```python
from build123d import *

# Parameters (mm, degrees)
RESSALTO_EXTRUS_O1_DEPTH   = 10
ESBO_O2_W                  = 10
ESBO_O2_H                  = 10
ESBO_O2_W_2                = 210
ESBO_O2_H_2                = 220
RESSALTO_EXTRUS_O4_DEPTH   = 50
ESBO_O7_R                  = 40
CORTE_EXTRUS_O1_DEPTH      = 3
ESBO_O21_W                 = 200
ESBO_O21_H                 = 25
CORTE_EXTRUS_O5_DEPTH      = 100
CORTE_EXTRUS_O6_DEPTH      = 161.25
CORTE_EXTRUS_O6_DEPTH_BACK = 1.25
ESBO_O23_W                 = 150
ESBO_O23_H                 = 5
RESSALTO_EXTRUS_O5_DEPTH   = 70


with BuildPart() as part:
    # Esboço1 → Ressalto-extrusão1 (new body)
    with BuildSketch(Plane.XY):
        Polygon((-99.217703787, 25.02394247), (70.782296213, 25.02394247), (70.782296213, 0), (70.782296213, -214.97605753), (-99.217703787, -214.97605753), (-269.217703787, -214.97605753), (-269.217703787, 0), (-269.217703787, 25.02394247), align=None)
    extrude(amount=RESSALTO_EXTRUS_O1_DEPTH)

    # Esboço2 → Ressalto-extrusão4 (add)
    with BuildSketch(Plane.XY.offset(10)):
        with Locations((-54.217703787, -209.97605753)):
            Rectangle(ESBO_O2_W, ESBO_O2_H)
        with Locations((-164.217703787, -209.97605753)):
            Rectangle(ESBO_O2_W_2, ESBO_O2_H)
        with Locations((-54.217703787, -94.97605753)):
            Rectangle(ESBO_O2_W, ESBO_O2_H_2)
        Polygon((-59.217703787, 15.02394247), (-49.217703787, 15.02394247), (-49.217703787, 25.02394247), (-269.217703787, 25.02394247), (-269.217703787, 15.02394247), align=None)
    extrude(amount=RESSALTO_EXTRUS_O4_DEPTH)

    # Esboço7 → Corte-extrusão1 (cut)
    with BuildSketch(Plane.XY.offset(10)):
        with Locations((10.782296213, -154.97605753)):
            Circle(ESBO_O7_R)
    extrude(amount=-CORTE_EXTRUS_O1_DEPTH, mode=Mode.SUBTRACT)

    # Esboço21 → Corte-extrusão5 (cut)
    with BuildSketch(Plane(origin=(0, 25.02394247, 0), x_dir=(1, 0, 0), z_dir=(0, 1, 0))):
        with Locations((-159.217703787, -37.5)):
            Rectangle(ESBO_O21_W, ESBO_O21_H)
    extrude(amount=-CORTE_EXTRUS_O5_DEPTH, mode=Mode.SUBTRACT)

    # Esboço23 → Corte-extrusão6 (cut, two sides: drawn at the far end of the back side and taken through both)
    with BuildSketch(Plane.XZ.offset(-15.02394247).offset(-CORTE_EXTRUS_O6_DEPTH_BACK)):
        with Locations((-194.217703787, 55)):
            Rectangle(ESBO_O23_W, ESBO_O23_H)
    extrude(amount=CORTE_EXTRUS_O6_DEPTH + CORTE_EXTRUS_O6_DEPTH_BACK, mode=Mode.SUBTRACT)

    # Esboço28 → Ressalto-extrusão5 (add)
    with BuildSketch(Plane.XY.offset(10)):
        Polygon((70.782296213, -84.97605753), (70.782296213, 25.02394247), (60.782296213, 25.02394247), (-39.217703787, 25.02394247), (-49.217703787, 25.02394247), (-49.217703787, -74.97605753), (-49.217703787, -84.97605753), align=None)
    extrude(amount=RESSALTO_EXTRUS_O5_DEPTH)


solid = part.part
```
Geometry check sheet. Reference: the model listing, model coordinates, mm. A direction names the side the tool comes from. Round coordinates to 2 decimals unless told otherwise and drop trailing zeros. Order: outer loops, then holes, each group sorted by start corner. A loop starts at its lowest first (then second) coordinate and runs counter-clockwise, first axis right, second up. Notation, with made-up numbers: M 39.25,61 L 69.25,61 A25 ccw 69.25,94 Z; hole C 79.25,28 d5. An arc over 180 degrees is marked long. Write item = value, one per line.
Q1. Release check for a two-part mould opening along X. For faces 6 (the flat face through (38, -120, 10)), 7 (the flat face through (-259.218, 20, 38)), 8 (the flat face through (-49.218, -29, 70)), 9 (the flat face through (10, -154, 7)) record: released by +X, released by -X, zero draft, split by the parting line, or undercut.
Answer block:
face_6 = zero draft
face_7 = undercut
face_8 = released by -X
face_9 = undercut
Q2. Set-up check for faces 1 (the flat face through (-163, -204.976, 35)), 2 (the flat face through (-49.218, -151, 35)), 3 (the cylindrical face through (5.575, -115.316, 8.521)), 4 (the flat face through (-161, 20, 50)), 5 (the flat face through (-54, -94, 60)): record each of +Z, -Z, +X, -X, +Y, -Y from which the full face is reachable in a straight line by a thin tool's end or side.
Answer block:
face_1 = +Z, -X
face_2 = +Z, +X, -Y
face_3 = +Z
face_4 = +Y
face_5 = +Z, -X, +Y, -Y
Q3. Scan lines: line 1 (Y direction, x = -135, z = 52); line 2 (Z direction, x = -44, y = -148.5); line 3 (X direction, y = -156, z = 21). Record each from-to range of solid material in increasing order.
Answer block:
line_1 = -214.98 to -204.98, 15.02 to 25.02
line_2 = 0 to 10
line_3 = -59.22 to -49.22
Q4. Section check A-A (z = 41). Enter the section's corners in (x, y), plus the area to 3 significant figures.
Answer block:
outline = M -269.22,-214.98 L -49.22,-214.98 L -49.22,-84.98 L 70.78,-84.98 L 70.78,25.02 L -59.22,25.02 L -59.22,-204.98 L -269.22,-204.98 Z; M -269.22,15.02 L -259.22,15.02 L -259.22,25.02 L -269.22,25.02 Z
area = 17,800 mm^2
Q5. Depth check by flat-ended pin: pin 1 Ø1 at (x, y) = (-201.5, 16) entering from +Z; pin 2 Ø2 at (y, z) = (-24.5, 32) entering from -X; pin 3 Ø25 at (y, z) = (-178, 29) entering from +X. Enter the tip coordinate at first touch or a pass-through.
Answer block:
pin_1 = 60
pin_2 = -59.22
pin_3 = -49.22
Q6. Section check B-B (x = -94.5). Enter the section's corners in (y, z), plus the area to 3 significant figures.
Answer block:
outline = M -214.98,0 L 25.02,0 L 25.02,25 L 15.02,25 L 15.02,10 L -204.98,10 L -204.98,60 L -214.98,60 Z; M 15.02,50 L 25.02,50 L 25.02,60 L 15.02,60 Z
area = 3,150 mm^2
Q7. Section check C-C (y = -69.5). Enter the section's corners in (x, z).
Answer block:
outline = M -269.22,0 L 70.78,0 L 70.78,80 L -49.22,80 L -49.22,60 L -59.22,60 L -59.22,10 L -269.22,10 Z
Q8. Section check D-D (z = 17.5). Enter the section's corners in (x, y).
Answer block:
outline = M -269.22,-214.98 L -49.22,-214.98 L -49.22,-84.98 L 70.78,-84.98 L 70.78,25.02 L -269.22,25.02 L -269.22,15.02 L -59.22,15.02 L -59.22,-204.98 L -269.22,-204.98 Z
